Print and shaded views of the part. All mm, measured from the part's lowest x, y and z. Coordinates: 2 decimals unless noted, no trailing zeros. Order: outer loops, then holes, each group sorted by start corner. A loop starts at its lowest first (then second) coordinate and runs counter-clockwise, first axis right, second up.
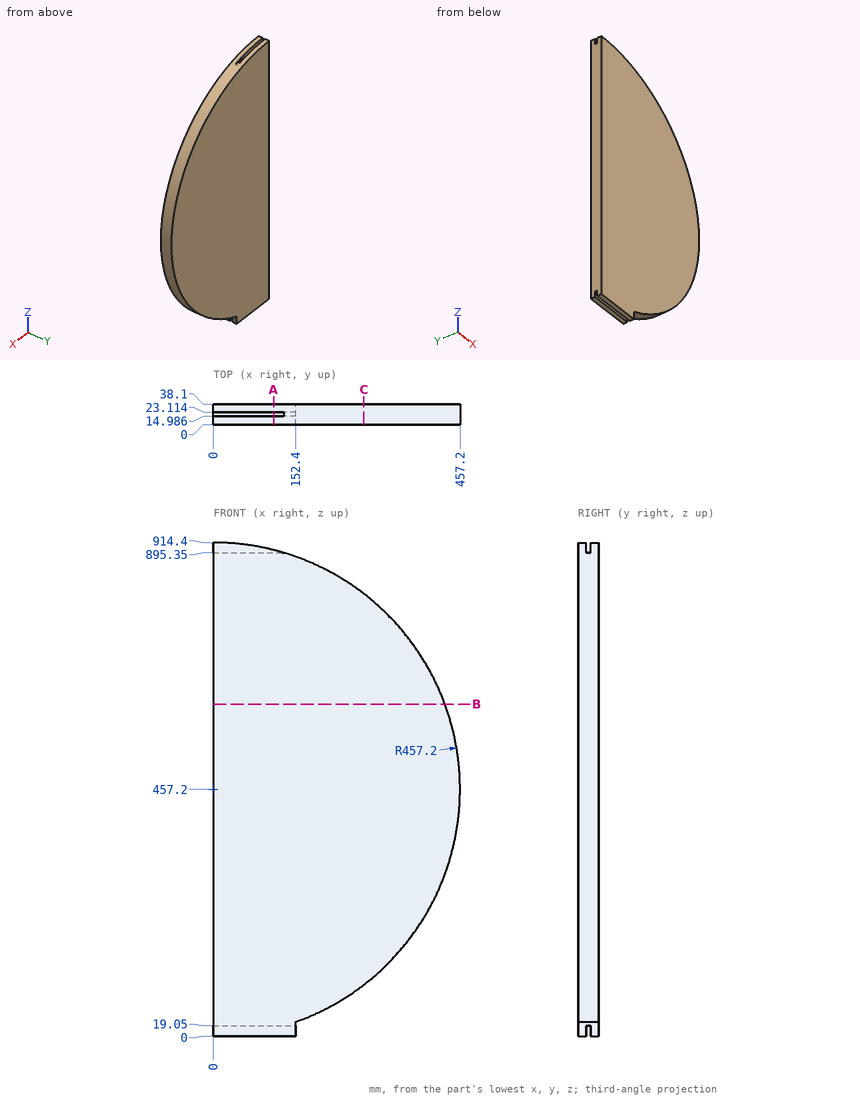
Q1. Cut at A-A, the plane x = 111.5. List the corners of the cut face in (y, z).
Established:
outline: (0, 0) - (14.99, 0) - (14.99, 19.05) - (23.11, 19.05) - (23.11, 0) - (38.1, 0) - (38.1, 900.6) - (23.11, 900.6) - (23.11, 895.35) - (14.99, 895.35) - (14.99, 900.6) - (0, 900.6) - close
Q2. Cut at B-B, the plane z = 615. List the corners of the cut face in (x, y).
Established:
outline: (0, 0) - (429.1, 0) - (429.1, 38.1) - (0, 38.1) - close
Q3. Probe line 1 (Z direction, x = 102, y = 23); line 2 (X direction, y = 11, z = 78.5); line 3 (X direction, y = 8.5, z = 134). List the from-to ranges inside material, lowest first.
Established:
line 1: z = 19.05 to 895.35
line 2: x = 0 to 256.16
line 3: x = 0 to 323.38
Q4. Cut at C-C, the plane x = 279. List the corners of the cut face in (y, z), plus the area to 3 significant figures.
Established:
outline: (0, 95) - (38.1, 95) - (38.1, 819.4) - (0, 819.4) - close
area: 27,600 mm2
Q5. Drop flat-ended pins along their axis: P1, Ø6, axis at x = 146, y = 17, coming from the +Z side; P2, Ø4, axis at x = 51, y = 17.5, coming from the +Z side. Give the stop position or say it passes through.
Established:
P1: stops at z = 891.46
P2: stops at z = 895.35
